Source: three-view drawing plus pictorial views. Frame: mm from the lowest corner of the part. Give positions to 0.01 mm unless a question says otherwise; leave off trailing zeros. Order: outer loops, then holes, each group sorted by start corner. A loop starts at its lowest first (then second) coordinate and runs counter-clockwise, first axis right, second up. Notation, with made-up numbers: M 55.25,63 L 84.25,63 A12 cw 84.25,74 Z; hole C 80.25,84.5 d6. An arc over 180 degrees is marked long. Use CSV: the item, a comma, the result in double quotes. Start each with the question number.
Item 1: Section query D-D on y = 713. Return loops of the section in (x, z).
Item 2: Section query B-B on y = 241. Return loops of the section in (x, z) (1 decimal).
Item 3: Section query C-C on x = 384. Return loops of the section in (y, z), and give its area (3 significant figures).
Item 4: Section query A-A on z = 216. Return loops of the section in (x, y).
Item 5: Ray query, probe 1 along X at (y, z) = (724.5, 182.5); probe 2 along Z at (x, y) = (479.5, 721.5); probe 3 along Y at (x, z) = (881.5, 473). Return the intervals inside material, ascending. Write a range as from..to.
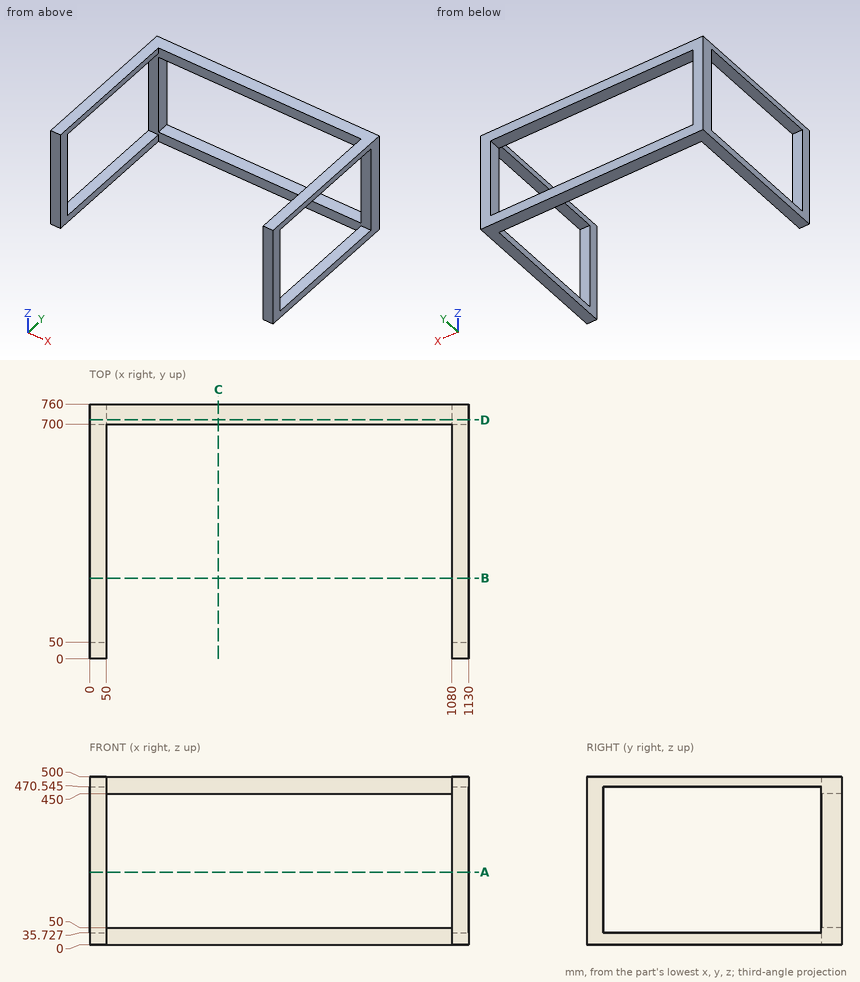
Verdict:
1,outline,"M 0,0 L 1130,0 L 1130,500 L 0,500 Z; hole M 50,50 L 1080,50 L 1080,450 L 50,450 Z"
2,outline,"M 0,0 L 50,0 L 50,35.7 L 0,35.7 Z; M 0,470.5 L 50,470.5 L 50,500 L 0,500 Z; M 1080,0 L 1130,0 L 1130,35.7 L 1080,35.7 Z; M 1080,470.5 L 1130,470.5 L 1130,500 L 1080,500 Z"
3,outline,"M 700,0 L 760,0 L 760,50 L 700,50 Z; M 700,450 L 760,450 L 760,500 L 700,500 Z"
3,area,"6,000 mm2"
4,outline,"M 0,0 L 50,0 L 50,50 L 0,50 Z; M 0,700 L 50,700 L 50,760 L 0,760 Z; M 1080,0 L 1130,0 L 1130,50 L 1080,50 Z; M 1080,700 L 1130,700 L 1130,760 L 1080,760 Z"
5,probe 1,"0..50, 1080..1130"
5,probe 2,"0..50, 450..500"
5,probe 3,"700..760"
